from build123d import *

# Parameters (mm, degrees)
F0_W     = 36.83
F0_H     = 40
F1_DEPTH = 55
F2_SIZE  = 29.21
F4_DEPTH = 35.56
F5_R     = 8.255
F6_DEPTH = 50.8


with BuildPart() as f1:
    # F0 (on Front) → F1 (new body)
    with BuildSketch(Plane.XZ):
        with Locations((18.415, 20)):
            Rectangle(F0_W, F0_H)
    extrude(amount=F1_DEPTH)

    # F2
    f2_edges = [f1.edges().sort_by_distance(p)[0] for p in [
        (18.415, -55, 40),
    ]]
    chamfer(f2_edges, length=F2_SIZE)

    # F3 (on face) → F4 (cut)
    with BuildSketch(Plane.XY.offset(40)):
        Polygon((29.21, 0), (7.62, 0), (7.62, -55.67665), (29.21, -55.354353), align=None)
    extrude(amount=-F4_DEPTH, mode=Mode.SUBTRACT)

    # F5 (on face) → F6 (cut)
    with BuildSketch(Plane.YZ.offset(36.83)):
        with Locations((-15.24, 21.59)):
            Circle(F5_R)
    extrude(amount=-F6_DEPTH, mode=Mode.SUBTRACT)


solid = f1.part
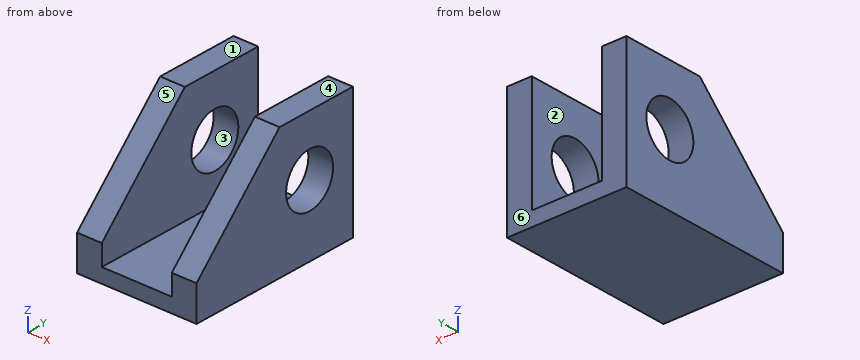
Read the model definition and answer for the solid it produces. Units are mm, in the model's axes. Face numbers are marked on the shaded views. A direction names the side the tool comes from. Give positions to 0.01 mm unless a question says otherwise; leave off trailing zeros. Loops run counter-clockwise (first coordinate to the right, second up) from the corner with the lowest first, then second, coordinate; pieces in that order, holes last. Notation, with made-up numbers: M -4,5.5 L 47,5.5 A17 cw 47,14.5 Z; hole C -32.5,-33.5 d8. An arc over 180 degrees is marked long. Write each question's results on one line, items separated by ' | '.
1. Given pin 1 (1.5 mm diameter, centred on x = 30, y = -6.5, fed in from -Z); pin 2 (4 mm diameter, centred on x = 19.5, y = -39.5, fed in from +Z), each flat-ended and moving along its own axis, determine where each tip first touches the part or whether it passes through.
Values:
pin 1: stops at z = 0 | pin 2: stops at z = 4.44
2. Straight lines are drawn through the part: line 1 (Z direction, x = 4, y = -15.24) (3 decimals); line 2 (X direction, y = -30, z = 21.5); line 3 (Z direction, x = 16.5, y = -42.5). For each, find the intervals that lie inside material, in ascending order. Write a range as [from, to].
Values:
line 1: z = [0, 13.335], [29.845, 40] | line 2: x = [0, 7.62], [29.21, 36.83] | line 3: z = [0, 4.44]
3. Section A-A on z = 21.59 is taken. Give the vertices of the cut face in (x, y) (3 decimals).
Values:
outline: M 0,-44.2 L 7.62,-44.2 L 7.62,-23.495 L 0,-23.495 Z; M 0,-6.985 L 7.62,-6.985 L 7.62,0 L 0,0 Z; M 29.21,-44.2 L 36.83,-44.2 L 36.83,-23.495 L 29.21,-23.495 Z; M 29.21,-6.985 L 36.83,-6.985 L 36.83,0 L 29.21,0 Z
4. Section C-C on x = 34.5 is taken. Give the vertices of the cut face in (y, z) (3 decimals).
Values:
outline: M -55,0 L 0,0 L 0,40 L -25.79,40 L -55,10.79 Z; hole C -15.24,21.59 d16.51
5. Section D-D on z = 8 is taken. Give the vertices of the cut face in (x, y).
Values:
outline: M 0,-55 L 7.62,-55 L 7.62,0 L 0,0 Z; M 29.21,-55 L 36.83,-55 L 36.83,0 L 29.21,0 Z
6. Section B-B on y = -15.24 is taken. Give the vertices of the cut face in (x, z) (3 decimals).
Values:
outline: M 0,0 L 36.83,0 L 36.83,13.335 L 29.21,13.335 L 29.21,4.44 L 7.62,4.44 L 7.62,13.335 L 0,13.335 Z; M 0,29.845 L 7.62,29.845 L 7.62,40 L 0,40 Z; M 29.21,29.845 L 36.83,29.845 L 36.83,40 L 29.21,40 Z
7. The mould has two halves that part along Y. Classify the marked faces 3, 4, 5 and 6: pulls with the +Y half, pulls with the -Y half, needs draft (parallel to the pull), parting line crosses it, or undercut.
Values:
face 3: undercut | face 4: needs draft | face 5: pulls with the -Y half | face 6: pulls with the +Y half
8. A tool of negligible diameter and unlimited length cuts with its end or side. For the marked faces 1 and 2, from which of +Z, -Z, +X, -X, +Y, -Y can it reach the whole face along a straight path? Write none if from no direction.
Values:
face 1: +Z, +X, -X, +Y, -Y | face 2: +Z, +Y, -Y
